The listing builds one solid part. Answer for the finished solid, in the listing's coordinates (mm). Coordinates: 2 decimals unless noted, no trailing zeros. Write each loop counter-clockwise with the first axis right and the second up, starting at its lowest first coordinate (ties: lowest second). Pieces come first, ordered by that corner, then holes.
(1) Straight lines are drawn through the part: line 1 (Y direction, x = 2.35, z = 0.5); line 2 (Z direction, x = 2.1, y = -56); line 3 (Z direction, x = 2.7, y = 5). For each, find the intervals that lie inside material, in ascending order.
(2) The part is cut by section B-B on x = 1.55. Give the number of separate pieces and of enclosed holes in the cut face, plus the area to 3 significant figures.
(3) Given P1, Ø2, axis at y = -31.46, z = -15.41, coming from the -X side; P2, Ø1.5, axis at x = 2.5, z = 19.5, coming from the +Y side, each flat-ended and moving along its own axis, determine where each tip first touches the part or whether it passes through.
(4) The part is cut by section D-D on z = -18.5. Determine the outline of the cut face in (x, y) (3 decimals), plus the area to 3 significant figures.
(5) The part is cut by section A-A on z = -3. Determine the outline of the cut face in (x, y).
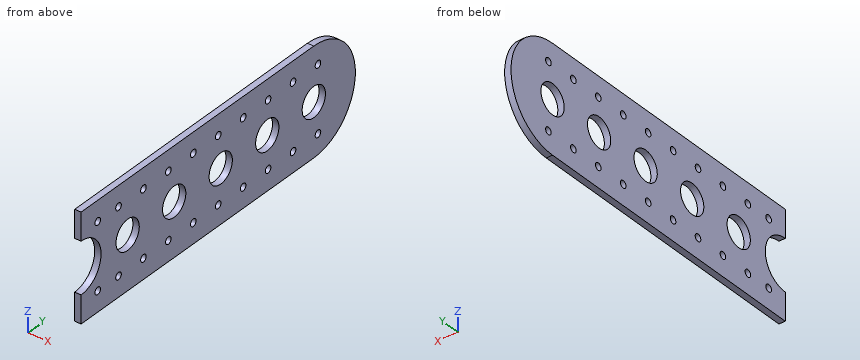
from build123d import *

# Parameters (mm, degrees)
SKETCH1_R           = 7.000001147
SKETCH1_R_2         = 6.999995031
SKETCH1_R_3         = 6.99997314
SKETCH1_R_4         = 6.999932994
SKETCH1_R_5         = 6.999971052
BOSS_EXTRUDE1_DEPTH = 3
SKETCH2_R           = 1.68
CUT_EXTRUDE3_DEPTH  = 88.676834918
SKETCH4_R           = 1.68
CUT_EXTRUDE4_DEPTH  = 88.676834918
LPATTERN2_COUNT     = 9
LPATTERN2_PITCH     = 15


with BuildPart() as part:
    # Sketch1 → Boss-Extrude1 (new body)
    with BuildSketch(Plane(origin=(0, 0, 0), x_dir=(0, 0, -1), z_dir=(1, 0, 0))):
        with BuildLine():
            Line((-25.094868708, -83.955196062), (-12.09486844, -83.955196062))
            ThreePointArc((-12.09486844, -83.955196062), (-0.094868335, -71.955195958), (11.905131769, -83.955196062))
            Line((11.905131769, -83.955196062), (24.905132037, -83.955196062))
            Line((24.905132037, -83.955196062), (24.905132037, 56.044804534))
            ThreePointArc((24.905132037, 56.044804534), (-0.094868335, 81.044804907), (-25.094868708, 56.044804534))
            Line((-25.094868708, 56.044804534), (-25.094868708, -83.955196062))
        make_face()
        with Locations((-0.094868335, -55.955176125)):
            Circle(SKETCH1_R, mode=Mode.SUBTRACT)
        with Locations((-0.094836539, -27.955201843)):
            Circle(SKETCH1_R_2, mode=Mode.SUBTRACT)
        with Locations((-0.094922892, 0.044802449)):
            Circle(SKETCH1_R_3, mode=Mode.SUBTRACT)
        with Locations((-0.094806508, 28.044865497)):
            Circle(SKETCH1_R_4, mode=Mode.SUBTRACT)
        with Locations((-0.094868335, 56.044746985)):
            Circle(SKETCH1_R_5, mode=Mode.SUBTRACT)
    extrude(amount=BOSS_EXTRUDE1_DEPTH)

    # Sketch2 → Cut-Extrude3 (cut, through all)
    with BuildSketch(Plane(origin=(3, 0, 0), x_dir=(0, 0, -1), z_dir=(1, 0, 0))):
        with Locations((-15.594868708, -73.955196062)):
            Circle(SKETCH2_R)
        with Locations((15.405132037, -73.955196062)):
            Circle(SKETCH2_R)
    extrude(amount=-CUT_EXTRUDE3_DEPTH, mode=Mode.SUBTRACT)

    # Sketch4 → Cut-Extrude4 (cut, through all)
    with BuildSketch(Plane(origin=(3, 0, 0), x_dir=(0, 0, -1), z_dir=(1, 0, 0))):
        with Locations((-15.594868708, -61.455196062)):
            Circle(SKETCH4_R)
        with Locations((15.405132037, -61.455196062)):
            Circle(SKETCH4_R)
    cut_extrude4 = extrude(amount=-CUT_EXTRUDE4_DEPTH, mode=Mode.SUBTRACT)

    # LPattern2: Cut-Extrude4 ×9
    with Locations(*[(0, i * LPATTERN2_PITCH, 0) for i in range(1, LPATTERN2_COUNT)]):
        add(cut_extrude4, mode=Mode.SUBTRACT)


solid = part.part
Model answer:
1. line 1: y = -71.96 to -62.94, -48.97 to -34.94, -20.97 to -6.94, 7.03 to 21.06, 35.03 to 49.06, 63.03 to 81.04
1. line 2: z = -24.91 to -6.9, 7.09 to 25.09
1. line 3: z = -24.91 to -4.85, 5.04 to 25.09
2. separate pieces: 1
2. enclosed holes: 25
2. area: 6,810 mm2
3. P1: passes through
3. P2: stops at y = 72.69
4. outline: (0, -83.955) - (3, -83.955) - (3, 72.755) - (0, 72.755) - close
4. area: 470 mm2
5. outline: (0, -72.36) - (3, -72.36) - (3, -62.23) - (0, -62.23) - close; (0, -49.68) - (3, -49.68) - (3, -34.23) - (0, -34.23) - close; (0, -21.68) - (3, -21.68) - (3, -6.23) - (0, -6.23) - close; (0, 6.32) - (3, 6.32) - (3, 21.77) - (0, 21.77) - close; (0, 34.32) - (3, 34.32) - (3, 49.77) - (0, 49.77) - close; (0, 62.32) - (3, 62.32) - (3, 80.85) - (0, 80.85) - close
